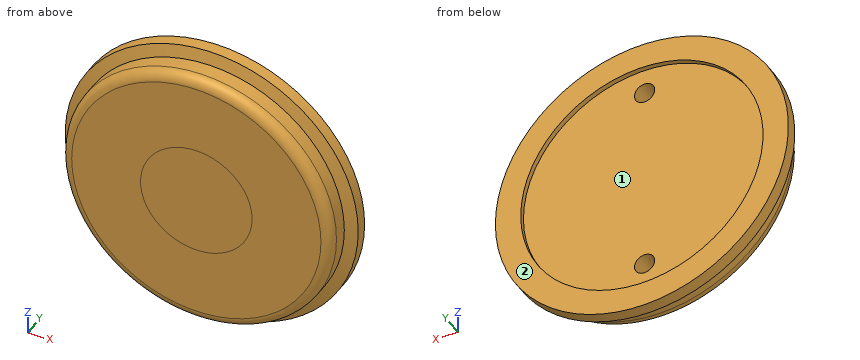
Autodesk Inventor part; units mm, degrees
ref_plane "YZ Plane" through (0, 0, 0) normal (1, 0, 0) x (0, 1, 0)
ref_plane "XZ Plane" through (0, 0, 0) normal (0, 1, 0) x (-1, 0, 0)
ref_plane "XY Plane" through (0, 0, 0) normal (0, 0, 1) x (1, 0, 0)
sketch "Sketch1" plane through (0, 0, 0) normal (0, 0, 1) x (1, 0, 0)
  line L0 (23.85, -0.0005) -> (46.0756, -0.0005)
  line L1 (46.0756, -0.0005) -> (46.0756, 12.7)
  line L2 (46.0756, 12.7) -> (0, 12.7)
  line L3 (0, 12.7) -> (0, 0)
  line L4 (17.5514, 12.7) -> (17.5514, -0.0005)
  line L5 (46.0756, 8.9662) -> (42.3672, 8.9662)
  line L6 (42.3672, 7.747) -> (42.3672, -0.0005)
  line L7 (46.0756, 7.747) -> (42.3672, 7.747)
  line L8 (46.0756, 8.9662) -> (42.3672, 7.747)
  line L9 (0, 11.1252) -> (0, 12.7)
  line L10 (17.5514, -0.0005) -> (23.85, -0.0005)
  line L11 (23.85, -0.0005) -> (23.85, -0.0005)
  line L12 (23.85, -0.0005) -> (0, -0.0005)
  line L13 (0, -0.0005) -> (0, 0)
  point P0 (17.5514, -0.0005)
  dimension "d0" = 46.0756
  dimension "d1" = 12.7
  dimension "d2" = 17.5514
  dimension "d3" = 3.7338
  dimension "d4" = 42.3672
  dimension "d6" = 4.953
  dimension "d14" = 23.85
  dimension "d15" = 0
revolve "Revolution1" add sketch "Sketch1" angle 360 about axis through (0, 12.7, 0) along (0, -1, 0) contours L10 L4 L2 L1 L8 L6 L0 | L12 L3 L2 L4
sketch "Sketch2" plane through (0, 12.7, 0) normal (0, 1, 0) x (1, 0, 0)
  circle A0 centre (0, 0) radius 38.1
  point P0 (0, 0)
  dimension "d11" = 76.2
extrude "Extrusion1" cut sketch "Sketch2" against normal blind 1.5748
sketch "Sketch5" plane through (0, 11.1252, 0) normal (0, 1, 0) x (1, 0, 0)
  circle A0 centre (0, 0) radius 30.1752
  point P0 (0, 0)
  point P1 (0, 30.1752)
  point P2 (0, -30.1752)
  dimension "d35" = 60.3504
hole "Hole3" at (0, 11.1252, -30.1752) at (0, 11.1252, 30.1752) direction (0, -1, 0) diameter 6.35 depth 7.62
fillet "Fillet1" radius 3.175 1 edges at (-42.3672, -0.0005, 0)
properties part number "2016.06.09 Mount Adapter Blank"
Verification items for the finished model (mm, model axes). Face numbers are marked on the shaded views. Give positions to 0.01 mm unless a question says otherwise; leave off trailing zeros. Order: outer loops, then holes, each group sorted by start corner. A loop starts at its lowest first (then second) coordinate and runs counter-clockwise, first axis right, second up. Notation, with made-up numbers: M 45,75 L 49,75 A26 ccw 49,107 Z; hole C 51.5,-15.5 d1. An arc over 180 degrees is marked long. Return JSON: item names as keys, results as strings. Group by question number.
1) Scan lines: line 1 (Z direction, x = 0, y = 12.4); line 2 (Z direction, x = 0, y = 7.5); line 3 (Y direction, x = -20.5, z = 19). Record each from-to range of solid material in increasing order.
2) Go/stop test with flat-tipped pins: pin 1 Ø1.5 at (y, z) = (5.5, -22.5) entering from +X; pin 2 Ø3 at (y, z) = (5, 16) entering from +X; pin 3 Ø4 at (x, z) = (0, -30.18) entering from +Y. Record where each tip stops, or that it passes through.
3) Mould release check, pull along Z, two halves, no side actions. Record for the marked faces 1 and 2: pulls with the +Z half, pulls with the -Z half, needs draft (parallel to the pull), parting line crosses it, or undercut.
4) Section check A-A on y = 2. Record the cut outline in (x, z).
Answer block:
{
 "1": {"line 1": "z = -46.08 to -38.1, 38.1 to 46.08", "line 2": "z = -42.37 to -33.35, -27 to 27, 33.35 to 42.37", "line 3": "y = 0 to 11.13"},
 "2": {"pin 1": "stops at x = 36.36", "pin 2": "stops at x = 39.81", "pin 3": "stops at y = 3.51"},
 "3": {"face 1": "undercut", "face 2": "needs draft"},
 "4": {"outline": "C 0,0 d84.28"}
}
